```python
from build123d import *

# Parameters (mm, degrees)
EXTRUDE_1_DEPTH = 0.7


with BuildPart() as part:
    # Sketch 288 → 拉伸1 (new body)
    with BuildSketch(Plane.XY):
        with BuildLine():
            Line((-0.6, -2.734958866), (-0.6, -3.484958866))
            ThreePointArc((-0.6, -3.484958866), (-1.2, -4.084958866), (-0.6, -4.684958866))
            Line((-0.6, -4.684958866), (-0.6, -5.284958866))
            ThreePointArc((-0.6, -5.284958866), (-1.652367602, -4.661606446), (-1.611408717, -3.439162917))
            ThreePointArc((-1.611408717, -3.439162917), (-1.582288686, -3.246338831), (-1.705946473, -3.095548061))
            ThreePointArc((-1.705946473, -3.095548061), (0, 4.1), (1.705946473, -3.095548061))
            ThreePointArc((1.705946473, -3.095548061), (1.582288686, -3.246338831), (1.611408717, -3.439162917))
            ThreePointArc((1.611408717, -3.439162917), (1.652367602, -4.661606446), (0.6, -5.284958866))
            Line((0.6, -5.284958866), (0.6, -4.684958866))
            ThreePointArc((0.6, -4.684958866), (1.2, -4.084958866), (0.6, -3.484958866))
            Line((0.6, -3.484958866), (0.6, -2.734958866))
            ThreePointArc((0.6, -2.734958866), (0, 2.8), (-0.6, -2.734958866))
        make_face()
    extrude(amount=EXTRUDE_1_DEPTH)


solid = part.part
```
Source: CAD feature listing. Evaluate the final solid. Frame: model axes, mm. Give positions to 0.01 mm unless a question says otherwise; leave off trailing zeros. Write each loop counter-clockwise with the first axis right and the second up, starting at its lowest first coordinate (ties: lowest second). Pieces come first, ordered by that corner, then holes. Notation, with made-up numbers: (55, 39) - (85, 39) arc R24 ccw to (85, 53) - close; hole circle Ø9 at (-29, 47). An arc over 180 degrees is marked (long way). One line per item, written item: value. Start each with the question number.
Q1. Material intervals for probe 1 along X at (y, z) = (0, 0.3); probe 2 along Y at (x, z) = (2.5, 0.15); probe 3 along X at (y, z) = (-3.25, 0.45), sorted ascending. Write a range as from..to.
Q2. Section query D-D, the plane x = 0. Return the cut outline in (y, z).
Q3. Section query C-C, the plane z = 0.1. Return the cut outline in (x, y), then the cut area to 3 significant figures.
Q4. Section query A-A, the plane y = 0. Return the cut outline in (x, z).
Q5. Section query B-B, the plane x = 1. Return the cut outline in (y, z), then the cut area to 3 significant figures.
Q6. Draft query along X for faces 1 (the face through (1.66, -4.65, 0.35)), 2 (the face through (1, 3, 0)), 3 (the face through (-0.1, 4.1, 0.3)), 4 (the face through (0.1, 2.8, 0.3)). Return one class per face: +X half, -X half, draft (parallel to the pull), parting line (faces both ways), or undercut.
Answer:
1. probe 1: x = -3.79..-2.8, 2.8..3.79
1. probe 2: y = -2.56..-1.26, 1.26..3.16
1. probe 3: x = -1.58..-0.6, 0.6..1.58
2. outline: (2.8, 0) - (4.1, 0) - (4.1, 0.7) - (2.8, 0.7) - close
3. outline: (-1.71, -3.1) arc R0.24 cw to (-1.61, -3.44) arc R1.2 ccw to (-0.6, -5.28) - (-0.6, -4.68) arc R0.6 cw to (-0.6, -3.48) - (-0.6, -2.73) arc R2.8 cw (long way) to (0.6, -2.73) - (0.6, -3.48) arc R0.6 cw to (0.6, -4.68) - (0.6, -5.28) arc R1.2 ccw to (1.61, -3.44) arc R0.24 cw to (1.71, -3.1) arc R3.8 ccw (long way) to start
3. area: 22.7 mm2
4. outline: (-3.79, 0) - (-2.8, 0) - (-2.8, 0.7) - (-3.79, 0.7) - close; (2.8, 0) - (3.79, 0) - (3.79, 0.7) - (2.8, 0.7) - close
5. outline: (-5.22, 0) - (-4.53, 0) - (-4.53, 0.7) - (-5.22, 0.7) - close; (-3.64, 0) - (-2.62, 0) - (-2.62, 0.7) - (-3.64, 0.7) - close; (2.62, 0) - (3.97, 0) - (3.97, 0.7) - (2.62, 0.7) - close
5. area: 2.14 mm2
6. face 1: +X half
6. face 2: draft
6. face 3: parting line
6. face 4: undercut
